Check sheet for the modelled part. Datum: model origin and axes. Units: mm. Face numbers are marked on the shaded views. Round coordinates to 2 decimals unless told otherwise and drop trailing zeros. Write each loop counter-clockwise with the first axis right and the second up, starting at its lowest first coordinate (ties: lowest second). Pieces come first, ordered by that corner, then holes.
Item 1: Release check for a two-part mould opening along Y. For the marked faces 1, 2, 3 and 4 record: pulls with the +Y half, pulls with the -Y half, needs draft (parallel to the pull), parting line crosses it, or undercut.
Item 2: Section check B-B, the plane z = 1.2. Record the cut outline in (x, y), plus the area to 3 significant figures.
Item 3: Section check D-D, the plane y = -6. Record the cut outline in (x, z), plus the area to 3 significant figures.
Item 4: Section check C-C, the plane x = 6.5. Record the cut outline in (y, z), plus the area to 3 significant figures.
Item 5: Material ranges on line 1 along X through (y, z) = (5.5, 1.7); line 2 along X through (y, z) = (-5, 1.35), recorded low to high.
Item 6: Section check A-A, the plane y = 0. Record the cut outline in (x, z).
from build123d import *

# Parameters (mm, degrees)
F0_R     = 1.33216
F0_R_2   = 3.5
F1_DEPTH = 2


with BuildPart() as f1:
    # F0 (on Top) → F1 (new body)
    with BuildSketch(Plane.XY):
        with BuildLine():
            ThreePointArc((-8.493127, -2.977716), (-3.535534, -3.535534), (-2.977716, -8.493127))
            ThreePointArc((-2.977716, -8.493127), (-2.607487, -8.614001), (-2.232376, -8.718744))
            ThreePointArc((-2.232376, -8.718744), (0, -7.722864), (2.232376, -8.718744))
            ThreePointArc((2.232376, -8.718744), (2.607487, -8.614001), (2.977716, -8.493127))
            ThreePointArc((2.977716, -8.493127), (3.535534, -3.535534), (8.493127, -2.977716))
            ThreePointArc((8.493127, -2.977716), (8.614001, -2.607487), (8.718744, -2.232376))
            ThreePointArc((8.718744, -2.232376), (7.722864, 0), (8.718744, 2.232376))
            ThreePointArc((8.718744, 2.232376), (8.614001, 2.607487), (8.493127, 2.977716))
            ThreePointArc((8.493127, 2.977716), (3.535534, 3.535534), (2.977716, 8.493127))
            ThreePointArc((2.977716, 8.493127), (2.607487, 8.614001), (2.232376, 8.718744))
            ThreePointArc((2.232376, 8.718744), (0, 7.722864), (-2.232376, 8.718744))
            ThreePointArc((-2.232376, 8.718744), (-2.607487, 8.614001), (-2.977716, 8.493127))
            ThreePointArc((-2.977716, 8.493127), (-3.535534, 3.535534), (-8.493127, 2.977716))
            ThreePointArc((-8.493127, 2.977716), (-8.614001, 2.607487), (-8.718744, 2.232376))
            ThreePointArc((-8.718744, 2.232376), (-7.722864, 0), (-8.718744, -2.232376))
            ThreePointArc((-8.718744, -2.232376), (-8.614001, -2.607487), (-8.493127, -2.977716))
        make_face()
        with Locations((0, -6)):
            Circle(F0_R, mode=Mode.SUBTRACT)
        with Locations((-6, 0)):
            Circle(F0_R, mode=Mode.SUBTRACT)
        Circle(F0_R_2, mode=Mode.SUBTRACT)
        with Locations((0, 6)):
            Circle(F0_R, mode=Mode.SUBTRACT)
        with Locations((6, 0)):
            Circle(F0_R, mode=Mode.SUBTRACT)
    extrude(amount=F1_DEPTH)


solid = f1.part
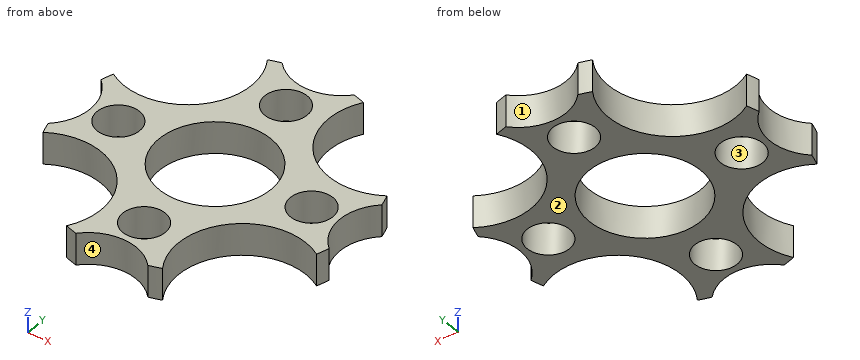
Values found:
1. face 1: pulls with the +Y half
1. face 2: needs draft
1. face 3: undercut
1. face 4: pulls with the -Y half
2. outline: (-8.72, -2.23) arc R9 ccw to (-8.49, -2.98) arc R4 cw to (-2.98, -8.49) arc R9 ccw to (-2.23, -8.72) arc R3 cw to (2.23, -8.72) arc R9 ccw to (2.98, -8.49) arc R4 cw to (8.49, -2.98) arc R9 ccw to (8.72, -2.23) arc R3 cw to (8.72, 2.23) arc R9 ccw to (8.49, 2.98) arc R4 cw to (2.98, 8.49) arc R9 ccw to (2.23, 8.72) arc R3 cw to (-2.23, 8.72) arc R9 ccw to (-2.98, 8.49) arc R4 cw to (-8.49, 2.98) arc R9 ccw to (-8.72, 2.23) arc R3 cw to start; hole circle Ø2.66 at (-6, 0); hole circle Ø7 at (0, 0); hole circle Ø2.66 at (0, -6); hole circle Ø2.66 at (0, 6); hole circle Ø2.66 at (6, 0)
2. area: 87.0 mm2
3. outline: (-2.38, 0) - (-1.33, 0) - (-1.33, 2) - (-2.38, 2) - close; (1.33, 0) - (2.38, 0) - (2.38, 2) - (1.33, 2) - close
3. area: 4.19 mm2
4. outline: (-2.37, 0) - (-1.23, 0) - (-1.23, 2) - (-2.37, 2) - close; (1.23, 0) - (2.37, 0) - (2.37, 2) - (1.23, 2) - close
4. area: 4.53 mm2
5. line 1: x = -2.46 to -1.23, 1.23 to 2.46
5. line 2: x = -2.6 to -0.88, 0.88 to 2.6
6. outline: (-7.72, 0) - (-7.33, 0) - (-7.33, 2) - (-7.72, 2) - close; (-4.67, 0) - (-3.5, 0) - (-3.5, 2) - (-4.67, 2) - close; (3.5, 0) - (4.67, 0) - (4.67, 2) - (3.5, 2) - close; (7.33, 0) - (7.72, 0) - (7.72, 2) - (7.33, 2) - close
